Autodesk Inventor part; units mm, degrees
ref_plane "YZ Plane" through (0, 0, 0) normal (1, 0, 0) x (0, 1, 0)
ref_plane "XZ Plane" through (0, 0, 0) normal (0, 1, 0) x (-1, 0, 0)
ref_plane "XY Plane" through (0, 0, 0) normal (0, 0, 1) x (1, 0, 0)
sketch "Sketch1" plane through (0, 0, 0) normal (0, 0, 1) x (1, 0, 0)
  circle A0 centre (-2.1414, -19.2098) radius 2
  circle A1 centre (-31.9098, -10.5586) radius 2
  circle A2 centre (6.5098, 10.5586) radius 2
  circle A3 centre (-23.2586, 19.2098) radius 2
  line L0 (-28.6845, 20.7851) -> (-21.6804, 24.6349)
  line L1 (-21.6804, 24.6349) -> (8.0851, 15.9845)
  line L2 (8.0851, 15.9845) -> (11.9349, 8.9804)
  line L3 (11.9349, 8.9804) -> (3.2845, -20.7851)
  line L4 (3.2845, -20.7851) -> (-3.7196, -24.6349)
  line L5 (-3.7196, -24.6349) -> (-33.4851, -15.9845)
  line L6 (-33.4851, -15.9845) -> (-37.3349, -8.9804)
  line L7 (-37.3349, -8.9804) -> (-28.6845, 20.7851)
  line L8 (9.5562, -25.8106) -> (19.9232, 9.8616)
  line L9 (19.9232, 9.8616) -> (13.1106, 22.2562)
  line L10 (13.1106, 22.2562) -> (-22.5616, 32.6232)
  line L11 (-22.5616, 32.6232) -> (-34.9562, 25.8106)
  line L12 (-34.9562, 25.8106) -> (-45.3232, -9.8616)
  line L13 (-45.3232, -9.8616) -> (-38.5106, -22.2562)
  line L14 (-38.5106, -22.2562) -> (-2.8384, -32.6232)
  line L15 (-2.8384, -32.6232) -> (9.5562, -25.8106)
  line L16 (-38.5106, -22.2562) -> (-165.5106, -22.2562)
  line L17 (-165.5106, -22.2562) -> (-165.5106, 34.8938)
  line L18 (-165.5106, 34.8938) -> (-38.5106, 34.8938)
  line L19 (-38.5106, 34.8938) -> (-38.5106, -22.2562)
  circle A4 centre (-12.7, 0) radius 11
  point P0 (0, 0)
  dimension "d0" = 127
  dimension "d1" = 57.15
  dimension "d2" = 57.15
extrude "Extrusion1" add sketch "Sketch1" along normal blind 6.35 contours L0 L1 L2 L3 L4 L5 L6 L7 | L15 L14 L19 L12 L11 L10 L9 L8 | L16 L17 L18 L19 L12 L13 | L13 L12 L19
sketch "Sketch2" plane through (0, 0, 0) normal (0, 0, -1) x (-1, 0, 0)
  line L0 (136.7986, -16.3493) -> (136.7986, -9.9993)
  line L1 (133.0902, -9.9993) -> (133.0902, -16.3493)
  line L2 (136.7986, 9.0507) -> (136.7986, 15.4007)
  line L3 (133.0902, 15.4007) -> (133.0902, 9.0507)
  line L4 (126.7402, -12.7) -> (130.4486, -12.7) construction
  line L5 (126.7402, 12.7) -> (130.4486, 12.7) construction
  circle A0 centre (128.5944, -12.7) radius 1.8542
  circle A1 centre (128.5944, 12.7) radius 1.8542
  dimension "d5" = 3.7084
  dimension "d6" = 3.7084
extrude "Extrusion2" cut sketch "Sketch2" against normal through all
sketch "Sketch3" plane through (0, 0, 0) normal (0, 0, -1) x (-1, 0, 0)
  line L0 (165.5106, 34.8938) -> (165.5106, -22.2562)
  line L1 (153.1125, 15.7309) -> (159.2102, 17.5031)
  line L2 (170.3558, -20.8481) -> (159.2102, 17.5031)
  line L3 (2.8384, -32.6232) -> (155.6197, 11.7778)
  line L4 (-9.5562, -25.8106) -> (2.8384, -32.6232)
  line L5 (-19.9232, 9.8616) -> (-9.5562, -25.8106)
  line L6 (-13.1106, 22.2562) -> (-19.9232, 9.8616)
  line L7 (154.986, 71.1081) -> (-13.1106, 22.2562)
  line L8 (145.7706, 63.7481) -> (155.0405, 31.851)
  line L9 (145.7706, 63.7481) -> (139.6729, 61.976)
  line L10 (139.6729, 61.976) -> (139.0916, 63.9761)
  line L11 (139.0916, 63.9761) -> (136.4086, 63.1964)
  line L12 (136.4086, 63.1964) -> (136.9899, 61.1963)
  line L13 (136.9899, 61.1963) -> (133.5752, 60.2039)
  line L14 (133.5752, 60.2039) -> (134.6101, 56.6429)
  line L15 (134.6101, 56.6429) -> (138.0248, 57.6352)
  line L16 (138.0248, 57.6352) -> (138.606, 55.6352)
  line L17 (138.606, 55.6352) -> (141.289, 56.4149)
  line L18 (141.289, 56.4149) -> (140.7078, 58.415)
  line L19 (140.7078, 58.415) -> (146.8055, 60.1871)
  line L20 (158.1753, 21.0641) -> (146.8055, 60.1871)
  line L21 (158.1753, 21.0641) -> (152.0776, 19.292)
  line L22 (152.0776, 19.292) -> (151.4964, 21.2921)
  line L23 (151.4964, 21.2921) -> (148.8134, 20.5123)
  line L24 (148.8134, 20.5123) -> (149.3946, 18.5123)
  line L25 (149.3946, 18.5123) -> (145.9799, 17.5199)
  line L26 (145.9799, 17.5199) -> (147.0148, 13.9588)
  line L27 (147.0148, 13.9588) -> (150.4295, 14.9512)
  line L28 (150.4295, 14.9512) -> (151.0108, 12.9512)
  line L29 (151.0108, 12.9512) -> (153.6938, 13.7309)
  line L30 (153.6938, 13.7309) -> (153.1125, 15.7309)
  circle A0 centre (132.6412, 48.0825) radius 1.8542
  circle A1 centre (139.7296, 23.6916) radius 1.8542
  circle A2 centre (2.1414, -19.2098) radius 2
  circle A3 centre (31.9098, -10.5586) radius 2
  circle A4 centre (-6.5098, 10.5586) radius 2
  circle A5 centre (23.2586, 19.2098) radius 2
  circle A6 centre (12.7, 0) radius 11
  point P0 (165.5106, -22.2562)
extrude "Extrusion3" [suppressed]
equation "\"d2\" = d1"
properties part number "tiltColumnStepperSide02" material "Gold"
Model file for the job. Use its own axes, mm. A direction names the side the tool comes from. Coordinates: 2 decimals unless noted, no trailing zeros. Write each loop counter-clockwise with the first axis right and the second up, starting at its lowest first coordinate (ties: lowest second). Pieces come first, ordered by that corner, then holes. Notation, with made-up numbers: (-23.75, 26.25) - (-2.75, 26.25) arc R18 cw to (-2.75, 56.25) - close; hole circle Ø10 at (88.5, 81.5). An arc over 180 degrees is marked (long way). Use a Markdown table: item, result. Add a question column.
Item 1: Band-saw the part on B-B, the plane x = -12.7. Write the cut outline in (y, z), and give its area (3 significant figures).
Item 2: 3-axis set-ups, long thin cutter, end or side, ignore diameter. For faces 5 (the face through (-28.672, 29.265, 3.131)), 6 (the face through (-101, -22.256, 3)), 7 (the face through (-74, 2, 6.35)): which of +Z, -Z, +X, -X, +Y, -Y reach the whole face in a straight line?
Item 3: Drop a flat-ended pin along its axis: pin 1 (3 mm diameter, centred on x = -2.14, y = -19.21, fed in from -Z). Give the stop position or say it passes through.
Item 4: Band-saw the part on C-C, the plane z = 4.75. Write the cut outline in (x, y), and give its area (3 significant figures).
Item 5: Band-saw the part on D-D, the plane x = -96. Write the cut outline in (y, z), and give its area (3 significant figures).
Item 6: Drill centre lines: line 1 along X through (y, z) = (-12, 6); line 2 along X through (y, z) = (11.5, 1.5); line 3 along Y through (x, z) = (-131, 4). Where is each one in solid material? Low to high.
Item 7: Band-saw the part on A-A, the plane y = 3. Write the cut outline in (x, z), and give its area (3 significant figures).
Item 8: Two-plate mould, pull along Y, no slides. Class faces 1 (the face through (14.67, -8.22, 3.13)), 2 (the face through (-2.539, 4.213, 3.131)), 3 (the face through (-165.511, 6, 3)), 4 (the face through (-33.908, -10.647, 3.131)): pulls with the +Y half, pulls with the -Y half, needs draft (parallel to the pull), parting line crosses it, or undercut.
A:
| question | item | result |
|---|---|---|
| 1 | outline | (-29.76, 0) - (-11, 0) - (-11, 6.35) - (-29.76, 6.35) - close; (11, 0) - (29.76, 0) - (29.76, 6.35) - (11, 6.35) - close |
| 1 | area | 238 mm² |
| 2 | face 5 | +Z, -Z, +Y |
| 2 | face 6 | +Z, -Z, -X, -Y |
| 2 | face 7 | +Z, +X, -X, +Y, -Y |
| 3 | pin 1 | passes through |
| 4 | outline | (-165.51, -22.26) - (-38.51, -22.26) - (-2.84, -32.62) - (9.56, -25.81) - (19.92, 9.86) - (13.11, 22.26) - (-22.56, 32.62) - (-34.96, 25.81) - (-38.51, 13.58) - (-38.51, 34.89) - (-165.51, 34.89) - close; hole circle Ø3.71 at (-128.59, -12.7); hole circle Ø3.71 at (-128.59, 12.7); hole circle Ø4 at (-31.91, -10.56); hole circle Ø4 at (-23.26, 19.21); hole circle Ø22 at (-12.7, 0); hole circle Ø4 at (-2.14, -19.21); hole circle Ø4 at (6.51, 10.56) |
| 4 | area | 9,750 mm² |
| 5 | outline | (-22.26, 0) - (34.89, 0) - (34.89, 6.35) - (-22.26, 6.35) - close |
| 5 | area | 363 mm² |
| 6 | line 1 | x = -165.51 to -130.31, -126.88 to -33.3, -30.52 to 13.57 |
| 6 | line 2 | x = -165.51 to -130.01, -127.18 to 4.75, 8.27 to 19.02 |
| 6 | line 3 | y = -22.26 to 34.89 |
| 7 | outline | (-165.51, 0) - (-23.28, 0) - (-23.28, 6.35) - (-165.51, 6.35) - close; (-2.12, 0) - (17.93, 0) - (17.93, 6.35) - (-2.12, 6.35) - close |
| 7 | area | 1,030 mm² |
| 8 | face 1 | pulls with the -Y half |
| 8 | face 2 | undercut |
| 8 | face 3 | needs draft |
| 8 | face 4 | undercut |
